```python
from build123d import *

# Parameters (mm, degrees)
STOCK_EXHAUST_M5_WASHER15_B_1_START         = 200
STOCK_EXHAUST_M5_WASHER15_B_1_OUTLINE_R     = 7.5
STOCK_EXHAUST_M5_WASHER15_B_1_DEPTH         = 15
STOCK_EXHAUST_M5_WASHER15_B_1_START_2       = 202
STOCK_EXHAUST_M5_WASHER15_B_1_2_OUTLINE_R   = 7.5
STOCK_EXHAUST_M5_WASHER15_B_1_2_OUTLINE_R_2 = 3
STOCK_EXHAUST_M5_WASHER15_B_1_2_DEPTH       = 13
SKETCH1_W                                   = 80
SKETCH1_H                                   = 40
BOSS_EXTRUDE1_DEPTH                         = 50
SKETCH2_W                                   = 21
SKETCH2_H                                   = 21
CUT_EXTRUDE1_DEPTH                          = 50
LPATTERN1_COUNT                             = 2
LPATTERN1_PITCH                             = 25
LPATTERN1_COL_COUNT                         = 2
LPATTERN1_COL_PITCH                         = 25


# Read off the part's stored shape, not the designer's step: Stock-Exhaust_M5_washer15_B-1
with BuildPart() as part:
    # Stock-Exhaust_M5_washer15_B-1 outline → Stock-Exhaust_M5_washer15_B-1 (new body)
    with BuildSketch(Plane.YZ.offset(STOCK_EXHAUST_M5_WASHER15_B_1_START)):
        Polygon((-40, -20), (-10, -20), (-10, -60), (30, -60), (30, -20), (60, -20), (60, 20), (30, 20), (30, 60), (-10, 60), (-10, 20), (-40, 20), align=None)
        with Locations((10, -50)):
            Circle(STOCK_EXHAUST_M5_WASHER15_B_1_OUTLINE_R, mode=Mode.SUBTRACT)
        with Locations((-23, 0)):
            Circle(STOCK_EXHAUST_M5_WASHER15_B_1_OUTLINE_R, mode=Mode.SUBTRACT)
        with Locations((43, 0)):
            Circle(STOCK_EXHAUST_M5_WASHER15_B_1_OUTLINE_R, mode=Mode.SUBTRACT)
        with Locations((10, 50)):
            Circle(STOCK_EXHAUST_M5_WASHER15_B_1_OUTLINE_R, mode=Mode.SUBTRACT)
    extrude(amount=STOCK_EXHAUST_M5_WASHER15_B_1_DEPTH)

    # Stock-Exhaust_M5_washer15_B-1 2 outline → Stock-Exhaust_M5_washer15_B-1 2 (add)
    # profile 1 of 4: a face of its own
    with BuildSketch(Plane.YZ.offset(STOCK_EXHAUST_M5_WASHER15_B_1_START_2)):
        with Locations((43, 0)):
            Circle(STOCK_EXHAUST_M5_WASHER15_B_1_2_OUTLINE_R)
        with Locations((43, 0)):
            Circle(STOCK_EXHAUST_M5_WASHER15_B_1_2_OUTLINE_R_2, mode=Mode.SUBTRACT)
    # profile 2 of 4: a face of its own
    with BuildSketch(Plane.YZ.offset(STOCK_EXHAUST_M5_WASHER15_B_1_START_2)):
        with Locations((10, 50)):
            Circle(STOCK_EXHAUST_M5_WASHER15_B_1_2_OUTLINE_R)
        with Locations((10, 50)):
            Circle(STOCK_EXHAUST_M5_WASHER15_B_1_2_OUTLINE_R_2, mode=Mode.SUBTRACT)
    # profile 3 of 4: a face of its own
    with BuildSketch(Plane.YZ.offset(STOCK_EXHAUST_M5_WASHER15_B_1_START_2)):
        with Locations((10, -50)):
            Circle(STOCK_EXHAUST_M5_WASHER15_B_1_2_OUTLINE_R)
        with Locations((10, -50)):
            Circle(STOCK_EXHAUST_M5_WASHER15_B_1_2_OUTLINE_R_2, mode=Mode.SUBTRACT)
    # profile 4 of 4: a face of its own
    with BuildSketch(Plane.YZ.offset(STOCK_EXHAUST_M5_WASHER15_B_1_START_2)):
        with Locations((-23, 0)):
            Circle(STOCK_EXHAUST_M5_WASHER15_B_1_2_OUTLINE_R)
        with Locations((-23, 0)):
            Circle(STOCK_EXHAUST_M5_WASHER15_B_1_2_OUTLINE_R_2, mode=Mode.SUBTRACT)
    extrude(amount=STOCK_EXHAUST_M5_WASHER15_B_1_2_DEPTH)

    # Sketch1 → Boss-Extrude1 (add)
    with BuildSketch(Plane.ZY.offset(-200)):
        with Locations((0, 10)):
            Rectangle(SKETCH1_W, SKETCH1_H)
    extrude(amount=BOSS_EXTRUDE1_DEPTH)

    # Sketch2 → Cut-Extrude1 (cut)
    with BuildSketch(Plane.ZY.offset(-150)):
        with Locations((0, 10)):
            Rectangle(SKETCH2_W, SKETCH2_H)
    cut_extrude1 = extrude(amount=-CUT_EXTRUDE1_DEPTH, mode=Mode.SUBTRACT)

    # LPattern1: Cut-Extrude1 ×2
    with Locations(*[(0, 0, i * LPATTERN1_PITCH) for i in range(1, LPATTERN1_COUNT)]):
        add(cut_extrude1, mode=Mode.SUBTRACT)

    # LPattern1 col: Cut-Extrude1 ×2
    with Locations(*[(0, 0, -i * LPATTERN1_COL_PITCH) for i in range(1, LPATTERN1_COL_COUNT)]):
        add(cut_extrude1, mode=Mode.SUBTRACT)


solid = part.part
```
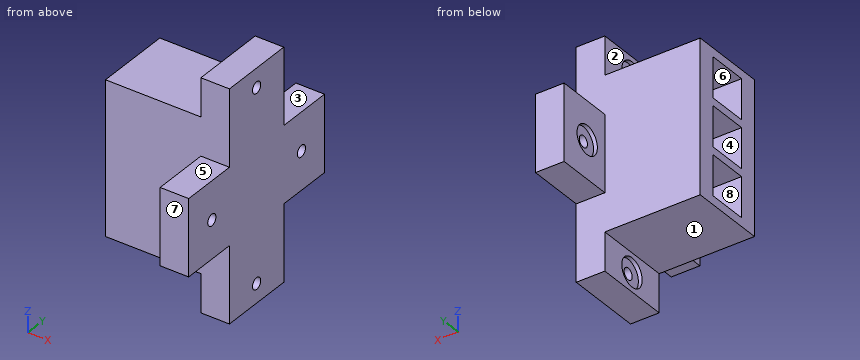
Check sheet for the modelled part. Datum: model origin and axes. Units: mm. Face numbers are marked on the shaded views. A direction names the side the tool comes from. Round coordinates to 2 decimals unless told otherwise and drop trailing zeros. Order: outer loops, then holes, each group sorted by start corner. A loop starts at its lowest first (then second) coordinate and runs counter-clockwise, first axis right, second up. Notation, with made-up numbers: (-28.75, 60.5) -> (25.25, 60.5) arc R15 ccw to (25.25, 80.5) -> close; hole circle Ø7 at (24, -4). An arc over 180 degrees is marked (long way). One line per item, written item: value. Start each with the question number.
Q1. Cross-section at A-A (z = 0). Record the boundary of the cut face in (x, y).
Q2. Set-up check for the marked faces 1, 2, 3 and 4: record each of +Z, -Z, +X, -X, +Y, -Y from which the full face is reachable in a straight line by a thin tool's end or side.
Q3. Mould release check, pull along Z, two halves, no side actions. Record for the marked faces 5, 6, 7 and 8: pulls with the +Z half, pulls with the -Z half, needs draft (parallel to the pull), parting line crosses it, or undercut.
Q4. Cross-section at D-D (y = 10). Give the number of separate pieces and of enclosed holes in the cut face, and give its area (3 significant figures).
Q5. Cross-section at B-B (z = -50). Record the boundary of the cut face in (x, y), and give its area (3 significant figures).
Q6. Gauge pin test, flat ends, axial feed: pin 1 Ø3.5 at (y, z) = (10, -50) entering from -X; pin 2 Ø7.5 at (x, y) = (210.5, 43) entering from +Z; pin 3 Ø6 at (x, z) = (160, -33) entering from +Y; pin 4 Ø6.5 at (x, y) = (172, 8) entering from -Z. Record the tip position at first contact, or that the pin passes through.
Q7. Cross-section at C-C (x = 162). Record the boundary of the cut face in (y, z), and give its area (3 significant figures).
Q8. Thickness scan on line 1 (Z direction, x = 200.6, y = 10); line 2 (Z direction, x = 205, y = 10); line 3 (Z direction, x = 175, y = 8). Record the ranges inside material, lowest first.
Completed:
1. outline: (150, -10) -> (200, -10) -> (200, -15.5) -> (202, -15.5) -> (202, -20) -> (215, -20) -> (215, 40) -> (202, 40) -> (202, 35.5) -> (200, 35.5) -> (200, 30) -> (150, 30) -> (150, 20.5) -> (200, 20.5) -> (200, -0.5) -> (150, -0.5) -> close; (200, -40) -> (215, -40) -> (215, -26) -> (202, -26) -> (202, -30.5) -> (200, -30.5) -> close; (200, 50.5) -> (202, 50.5) -> (202, 46) -> (215, 46) -> (215, 60) -> (200, 60) -> close
2. face 1: -Z, -X, +Y, -Y
2. face 2: +Z, -X, +Y, -Y
2. face 3: +Z, +X, -X, +Y
2. face 4: -X
3. face 5: pulls with the +Z half
3. face 6: undercut
3. face 7: needs draft
3. face 8: undercut
4. separate pieces: 3
4. enclosed holes: 0
4. area: 2,430 mm²
5. outline: (200, -10) -> (215, -10) -> (215, 7) -> (202, 7) -> (202, 2.5) -> (200, 2.5) -> close; (200, 17.5) -> (202, 17.5) -> (202, 13) -> (215, 13) -> (215, 30) -> (200, 30) -> close
5. area: 492 mm²
6. pin 1: passes through
6. pin 2: stops at z = 20
6. pin 3: stops at y = 30
6. pin 4: stops at z = -40
7. outline: (-10, -40) -> (30, -40) -> (30, 40) -> (-10, 40) -> close; hole (-0.5, -35.5) -> (20.5, -35.5) -> (20.5, -14.5) -> (-0.5, -14.5) -> close; hole (-0.5, -10.5) -> (20.5, -10.5) -> (20.5, 10.5) -> (-0.5, 10.5) -> close; hole (-0.5, 14.5) -> (20.5, 14.5) -> (20.5, 35.5) -> (-0.5, 35.5) -> close
7. area: 1,880 mm²
8. line 1: z = -60 to -57.5, -42.5 to 42.5, 57.5 to 60
8. line 2: z = -60 to -53, -47 to 47, 53 to 60
8. line 3: z = -40 to -35.5, -14.5 to -10.5, 10.5 to 14.5, 35.5 to 40
